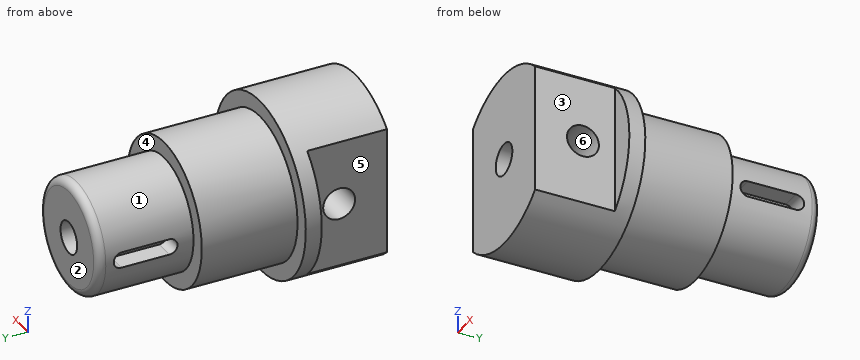
from build123d import *

# Parameters (mm, degrees)
CUT_EXTRUDE1_DEPTH = 20
CUT_EXTRUDE2_START = 9
CUT_EXTRUDE2_DEPTH = 20
HOLE1_D            = 8
FILLET1_R          = 2


with BuildPart() as part:
    # Sketch1 → Revolve1 (revolve)
    with BuildSketch(Plane.XY, mode=Mode.PRIVATE) as revolve1_sk:
        Polygon((4, 0), (4, 72), (14, 72), (14, 48), (18, 48), (18, 24), (22, 24), (22, 0), align=None)
    revolve(revolve1_sk.sketch.rotate(Axis((0, 0, 0), (0, 1, 0)), 90), axis=Axis((0, 0, 0), (0, 1, 0)))

    # Sketch2 → Cut-Extrude1 (cut)
    with BuildSketch(Plane.XZ):
        with BuildLine():
            Line((15, 16.093476939), (15, -16.093476939))
            ThreePointArc((15, -16.093476939), (22, 0), (15, 16.093476939))
        make_face()
    cut_extrude1 = extrude(amount=-CUT_EXTRUDE1_DEPTH, mode=Mode.SUBTRACT)

    # Sketch3 → Cut-Extrude2 (cut)
    with BuildSketch(Plane(origin=(0, 0, 0), x_dir=(0, 0, -1), z_dir=(1, 0, 0)).offset(CUT_EXTRUDE2_START)):
        with BuildLine():
            Line((2, 66), (2, 54))
            ThreePointArc((2, 54), (0, 52), (-2, 54))
            Line((-2, 54), (-2, 66))
            ThreePointArc((-2, 66), (0, 68), (2, 66))
        make_face()
    cut_extrude2 = extrude(amount=CUT_EXTRUDE2_DEPTH, mode=Mode.SUBTRACT)

    # Hole1 (through all)
    with Locations(Plane(origin=(15, 0, 0), x_dir=(0, 0, -1), z_dir=(1, 0, 0))):
        with Locations((0, 12)):
            Hole(HOLE1_D / 2)

    # Mirror2: Cut-Extrude2 across plane
    add(cut_extrude2.mirror(Plane(origin=(0, 0, 0), x_dir=(0, 0, 1), z_dir=(1, 0, 0))), mode=Mode.SUBTRACT)

    # Mirror3: Cut-Extrude1 across plane
    add(cut_extrude1.mirror(Plane(origin=(0, 0, 0), x_dir=(0, 0, 1), z_dir=(1, 0, 0))), mode=Mode.SUBTRACT)

    # Fillet1
    fillet1_edges = [part.edges().sort_by_distance(p)[0] for p in [
        (0, 72, 14),
    ]]
    fillet(fillet1_edges, radius=FILLET1_R)


solid = part.part
Read the model definition and answer for the solid it produces. Units are mm, in the model's axes. Face numbers are marked on the shaded views. A direction names the side the tool comes from. Give positions to 0.01 mm unless a question says otherwise; leave off trailing zeros. Write each loop counter-clockwise with the first axis right and the second up, starting at its lowest first coordinate (ties: lowest second). Pieces come first, ordered by that corner, then holes. Notation, with made-up numbers: (11, 1) - (61, 1) arc R29 ccw to (61, 31) - close; hole circle Ø6 at (-25.5, -38). An arc over 180 degrees is marked (long way). Return JSON: item names as keys, results as strings.
Q1. Given P1, Ø5.5, axis at x = -18.5, z = 3.5, coming from the -Y side; P2, Ø5.5, axis at x = -10.5, y = 59, coming from the +Z side; P3, Ø4, axis at x = -13, y = 31, coming from the +Z side; P4, Ø7.5, axis at x = 17.5, z = 0, coming from the -Y side, each flat-ended and moving along its own axis, determine where each tip first touches the part or whether it passes through.
Reply:
{"P1": "y = 20", "P2": "z = 11.66", "P3": "z = 14.25", "P4": "y = 0"}
Q2. Consider line 1 along X through (y, z) = (56, 0); line 2 along X through (y, z) = (51, 0); line 3 along Y through (x, z) = (-10, 19.5). Determine where each line is inside the solid, lowest interval first. Write a range as [from, to].
Reply:
{"line 1": "[-9, -4], [4, 9]", "line 2": "[-14, -4], [4, 14]", "line 3": "[0, 24]"}
Q3. A cutting plane is placed at A-A, the plane y = 56. Determine the outline of the cut face in (x, z).
Reply:
{"outline": "(-13.86, -2) arc R14 ccw to (13.86, -2) - (9, -2) - (9, 2) - (13.86, 2) arc R14 ccw to (-13.86, 2) - (-9, 2) - (-9, -2) - close; hole circle Ø8 at (0, 0)"}
Q4. A cutting plane is placed at B-B, the plane x = 16.5. Determine the outline of the cut face in (y, z).
Reply:
{"outline": "(20, -14.55) - (24, -14.55) - (24, -7.19) - (48, -7.19) - (48, 7.19) - (24, 7.19) - (24, 14.55) - (20, 14.55) - close"}
Q5. For the marked faces 1, 2 and 3, determine the directions among +Z, -Z, +X, -X, +Y, -Y from which every point of the face is accessible in a straight line to the end or side of a thin tool.
Reply:
{"face 1": "+Y", "face 2": "+Z, -Z, +X, -X, +Y", "face 3": "+Z, -Z, +X, -Y"}
Q6. For a pull along Y with two mould halves and no side action, classify the marked faces 4, 5 and 6 as released by +Y, released by -Y, zero draft, split by the parting line, or undercut.
Reply:
{"face 4": "released by +Y", "face 5": "zero draft", "face 6": "undercut"}
Q7. A cutting plane is placed at C-C, the plane x = -10. Count the separate pieces of the cut face and the enclosed holes in it, and give its area (3 significant figures).
Reply:
{"separate pieces": "1", "enclosed holes": "2", "area": "2,020 mm²"}
